```python
from build123d import *

# Parameters (mm, degrees)
PAD_DEPTH    = 45
SKETCH001_R  = 12
POCKET_DEPTH = 160.001
FILLET_R     = 8


with BuildPart() as part:
    # Sketch → Pad (new body)
    with BuildSketch(Plane.XY):
        with BuildLine():
            ThreePointArc((-30, 0), (-50, 20), (-70, 0))
            Line((-70, 0), (-70, -40))
            Line((-70, -40), (-80, -40))
            Line((-80, 40), (-80, -40))
            Line((80, 40), (-80, 40))
            Line((80, -40), (80, 40))
            Line((70, -40), (80, -40))
            Line((70, 0), (70, -40))
            ThreePointArc((70, 0), (49.999978, 20), (30, -4.5e-05))
            Line((30, -4.5e-05), (30, -40.000045))
            Line((20, -40.000045), (30, -40.000045))
            Line((20, -4.5e-05), (20, -40.000045))
            ThreePointArc((20, -4.5e-05), (2.2e-05, 20), (-20, 0))
            Line((-20, 0), (-20, -40))
            Line((-30, -40), (-20, -40))
            Line((-30, 0), (-30, -40))
        make_face()
    extrude(amount=PAD_DEPTH)

    # Sketch001 → Pocket (cut, through all)
    with BuildSketch(Plane(origin=(-80, 0, 0), x_dir=(0, -1, 0), z_dir=(-1, 0, 0))):
        with Locations((-40, 22.5)):
            Circle(SKETCH001_R)
    extrude(amount=-POCKET_DEPTH, mode=Mode.SUBTRACT)

    # Fillet
    fillet_edges = [part.edges().sort_by_distance(p)[0] for p in [
        (0, 40, 34.5),
        (0, 40, 10.5),
    ]]
    fillet(fillet_edges, radius=FILLET_R)


solid = part.part
```
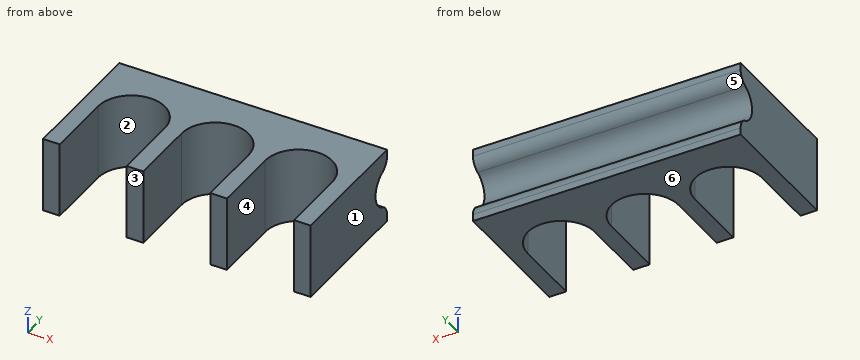
Design review of the part built by this model. Coordinates are the model's own, in mm. Face numbers are marked on the shaded views. A direction names the side the tool comes from. Coordinates: 2 decimals unless noted, no trailing zeros. Loops run counter-clockwise (first coordinate to the right, second up) from the corner with the lowest first, then second, coordinate; pieces in that order, holes last. Notation, with made-up numbers: (-5, -7) -> (27, -7) arc R19 cw to (27, -2) -> close; hole circle Ø8 at (17, 11). An arc over 180 degrees is marked (long way). Answer as a JSON object with one key per item and string values.
Q1. Take a section at D-D on z = 24. Give the boundary of the cut face in (x, y).
Answer block:
{"outline": "(-80, -40) -> (-70, -40) -> (-70, 0) arc R20 cw to (-30, 0) -> (-30, -40) -> (-20, -40) -> (-20, 0) arc R20 cw to (20, 0) -> (20, -40) -> (30, -40) -> (30, 0) arc R20 cw to (70, 0) -> (70, -40) -> (80, -40) -> (80, 28.09) -> (-80, 28.09) -> close"}
Q2. Take a section at C-C on z = 13.5. Give the boundary of the cut face in (x, y).
Answer block:
{"outline": "(-80, -40) -> (-70, -40) -> (-70, 0) arc R20 cw to (-30, 0) -> (-30, -40) -> (-20, -40) -> (-20, 0) arc R20 cw to (20, 0) -> (20, -40) -> (30, -40) -> (30, 0) arc R20 cw to (70, 0) -> (70, -40) -> (80, -40) -> (80, 32.06) -> (-80, 32.06) -> close"}
Q3. Take a section at B-B on x = -50. Give the boundary of the cut face in (y, z).
Answer block:
{"outline": "(20, 0) -> (40, 0) -> (40, 4.17) arc R8 ccw to (35.2, 11.5) arc R12 cw to (35.2, 33.5) arc R8 ccw to (40, 40.83) -> (40, 45) -> (20, 45) -> close"}
Q4. The part is to be moulded in two halves that separate along X. For the marked faces 1, 2 and 3, say which applies: +X half, -X half, draft (parallel to the pull), parting line (faces both ways), or undercut.
Answer block:
{"face 1": "+X half", "face 2": "undercut", "face 3": "draft"}
Q5. Tool access review of the marked faces 4, 5 and 6: name each direction out of +Z, -Z, +X, -X, +Y, -Y from which nothing blocks a thin tool from reaching the whole face with its end or side.
Answer block:
{"face 4": "+Z, -Z, -Y", "face 5": "+X, -X, +Y", "face 6": "-Z, +X, -X, +Y, -Y"}
Q6. To check wall thickness, follow L1, parallel to X at y = -25, z = 34; L2, parallel to X at y = 9.5, z = 2; L3, parallel to Y at x = -26.5, z = 22.5. State the ranges of each line that lie inside material, in increasing order.
Answer block:
{"L1": "x = -80 to -70, -30 to -20, 20 to 30, 70 to 80", "L2": "x = -80 to -67.6, -32.4 to -17.6, 17.6 to 32.4, 67.6 to 80", "L3": "y = -40 to 28"}
Q7. Clearance check with flat-ended pins moving along their axes: pin 1 Ø8 at (x, z) = (-9, 13) entering from +Y; pin 2 Ø8 at (x, z) = (-0.5, 22) entering from -Y; pin 3 Ø4 at (x, z) = (-4.5, 22.5) entering from +Y. State where each tip first meets the part, or that it passes through.
Answer block:
{"pin 1": "stops at y = 38.38", "pin 2": "stops at y = 19.49", "pin 3": "stops at y = 28.17"}
Q8. Take a section at A-A on y = -24. Give the boundary of the cut face in (x, z).
Answer block:
{"outline": "(-80, 0) -> (-70, 0) -> (-70, 45) -> (-80, 45) -> close; (-30, 0) -> (-20, 0) -> (-20, 45) -> (-30, 45) -> close; (20, 0) -> (30, 0) -> (30, 45) -> (20, 45) -> close; (70, 0) -> (80, 0) -> (80, 45) -> (70, 45) -> close"}
